Here's how the part is built. I have some questions about the finished solid (model axes, mm). Face numbers are marked on the shaded views. A direction names the side the tool comes from. Round coordinates to 2 decimals unless told otherwise and drop trailing zeros. Put each result on its own line as item: value. Start each with the question number.
1) Will these pins go through, and if not, where does the flat tip stop? P1, Ø3.5, axis at x = -4.95, z = 4.95, coming from the -Y side; P2, Ø3.5, axis at x = -4.95, z = -4.95, coming from the +Y side; P3, Ø1, axis at x = -5, y = 24, coming from the +Z side.
2) Which directions (+Z, -Z, +X, -X, +Y, -Y) give clear straight access to the entire face, cutting with the end or side of a thin tool? Please do the marked faces 1 and 2.
3) If I drill on line 1 along Y through (x, z) = (-8.5, -6.25); line 2 along Z through (x, y) = (12, 13); line 3 along Y through (x, z) = (-2, 2.75), over which ranges is the centre line in solid material (lowest first)? Write a range as [from, to].
from build123d import *

# Parameters (mm, degrees)
FILLET1_R                = 1.5
BOSS_EXTRUDE1_DEPTH      = 4.45
BOSS_EXTRUDE1_DEPTH_BACK = 0.25
SKETCH3_R                = 12
FILLET2_R                = 1
SKETCH4_R                = 10
CUT_EXTRUDE1_DEPTH       = 2.45
SKETCH8_R                = 1.1
CUT_EXTRUDE2_DEPTH       = 38.80294317
CIRPATTERN1_COUNT        = 4


with BuildPart() as part:
    # Sketch1 → Loft1 section 0
    with BuildSketch(Plane(origin=(0, 0, 0), x_dir=(1, 0, 0), z_dir=(0, 1, 0))):
        with BuildLine():
            Line((-20, 1.5), (20, 1.5))
            Line((20, 1.5), (20, -1.5))
            Line((20, -1.5), (-20, -1.5))
            Line((-20, -1.5), (-20, 1.5))
        make_face()
    # Sketch2 → Loft1 section 1
    with BuildSketch(Plane(origin=(0, 30, 0), x_dir=(1, 0, 0), z_dir=(0, 1, 0))):
        with BuildLine():
            Line((-12.5, 1.5), (12.5, 1.5))
            Line((12.5, 1.5), (12.5, -1.5))
            Line((12.5, -1.5), (-12.5, -1.5))
            Line((-12.5, -1.5), (-12.5, 1.5))
        make_face()
    loft()

    # Fillet1
    fillet1_edges = [part.edges().sort_by_distance(p)[0] for p in [
        (0, 30, -1.5),
        (-12.5, 30, 0),
        (0, 30, 1.5),
        (12.5, 30, 0),
        (16.25, 15, 1.5),
        (-16.25, 15, 1.5),
        (16.25, 15, -1.5),
        (-16.25, 15, -1.5),
    ]]
    fillet(fillet1_edges, radius=FILLET1_R - 0.0001)  # a hair under: the kernel refuses the full size

    # Sketch3 → Boss-Extrude1 (add, two sides: drawn at the far end of the back side and taken through both)
    with BuildSketch(Plane.XZ.offset(-BOSS_EXTRUDE1_DEPTH_BACK)):
        with Locations(Location((0, 0, 0), (0, 0, 270))):
            Circle(SKETCH3_R)
    extrude(amount=BOSS_EXTRUDE1_DEPTH + BOSS_EXTRUDE1_DEPTH_BACK)

    # Fillet2
    fillet2_edges = [part.edges().sort_by_distance(p)[0] for p in [
        (0, 0.25, 1.5),
        (0, 0.25, -1.5),
        (0, -4.45, 12),
    ]]
    fillet(fillet2_edges, radius=FILLET2_R)

    # Sketch4 → Cut-Extrude1 (cut)
    with BuildSketch(Plane.XZ.offset(4.45)):
        with Locations(Location((0, 0, 0), (0, 0, 270))):
            Circle(SKETCH4_R)
    extrude(amount=-CUT_EXTRUDE1_DEPTH, mode=Mode.SUBTRACT)

    # Sketch8 → Cut-Extrude2 (cut, through all)
    with BuildSketch(Plane(origin=(0, 0.25, 0), x_dir=(1, 0, 0), z_dir=(0, 1, 0))):
        with Locations(Location((4.949747468, 4.949747468, 0), (0, 0, 270))):
            Circle(SKETCH8_R)
    cut_extrude2 = extrude(amount=-CUT_EXTRUDE2_DEPTH, mode=Mode.SUBTRACT)

    # CirPattern1: Cut-Extrude2 ×4 about axis
    cirpattern1_axis = Axis((0, 0, 0), (0, 1, 0))
    for i in range(1, CIRPATTERN1_COUNT):
        add(cut_extrude2.rotate(cirpattern1_axis, i * 360 / CIRPATTERN1_COUNT), mode=Mode.SUBTRACT)


solid = part.part
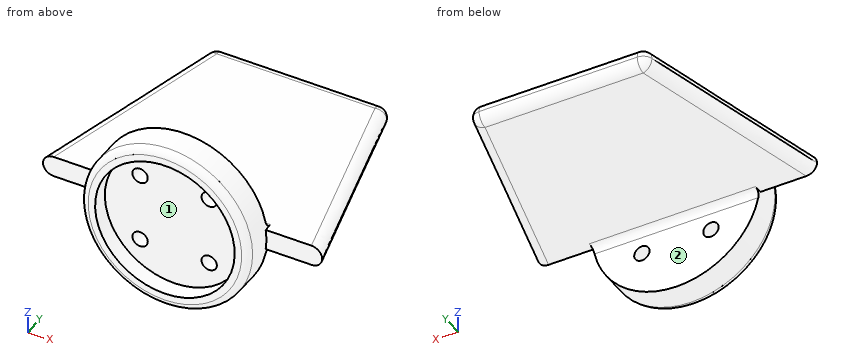
Findings:
1. P1: stops at y = -2
1. P2: stops at y = 0.25
1. P3: stops at z = 1.5
2. face 1: -Y
2. face 2: -Z, +X, -X, +Y
3. line 1: y = [-4.45, 0.25]
3. line 2: z = [-1.5, 1.5]
3. line 3: y = [-2, 0.25]
